Input: part model. Units: mm. Frame: model coordinates. Face numbers are marked on the shaded views. A direction names the side the tool comes from. Coordinates: 2 decimals unless noted, no trailing zeros. Order: outer loops, then holes, each group sorted by start corner. A loop starts at its lowest first (then second) coordinate and runs counter-clockwise, first axis right, second up. Notation, with made-up numbers: (38, -21.5) - (46, -21.5) arc R27 ccw to (46, 5.5) - close; hole circle Ø2 at (33.25, -26). An arc over 180 degrees is marked (long way). Use a Markdown table: item, result. Add a question column.
from build123d import *

# Parameters (mm, degrees)
SKETCH1_R           = 4
BOSS_EXTRUDE1_DEPTH = 1
SKETCH2_R           = 3
BOSS_EXTRUDE2_DEPTH = 2
FILLET1_R           = 1
SKETCH3_R           = 2
CUT_EXTRUDE1_DEPTH  = 4
FILLET2_R           = 1


with BuildPart() as part:
    # Sketch1 → Boss-Extrude1 (new body)
    with BuildSketch(Plane.XY):
        Circle(SKETCH1_R)
    extrude(amount=BOSS_EXTRUDE1_DEPTH)

    # Sketch2 → Boss-Extrude2 (add)
    with BuildSketch(Plane.XY.offset(1)):
        Circle(SKETCH2_R)
    extrude(amount=BOSS_EXTRUDE2_DEPTH)

    # Fillet1
    fillet1_edges = [part.edges().sort_by_distance(p)[0] for p in [
        (-3, 0, 1),
    ]]
    fillet(fillet1_edges, radius=FILLET1_R - 0.0001)  # a hair under: the kernel refuses the full size

    # Sketch3 → Cut-Extrude1 (cut)
    with BuildSketch(Plane.XY.offset(3)):
        Circle(SKETCH3_R)
    extrude(amount=-CUT_EXTRUDE1_DEPTH, mode=Mode.SUBTRACT)

    # Fillet2
    fillet2_edges = [part.edges().sort_by_distance(p)[0] for p in [
        (-2, 0, 0),
    ]]
    fillet(fillet2_edges, radius=FILLET2_R)


solid = part.part
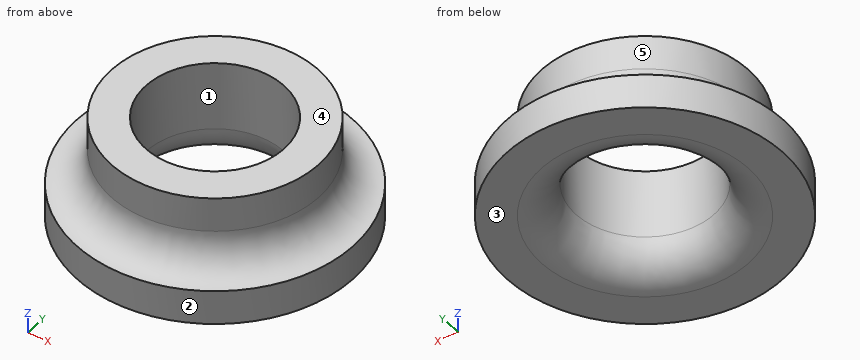
1) Cut plane D-D (z = 0.4). Return the cut outline in (x, y), and give its area (3 significant figures).
2) Contact query for a flat-ended pin moving along its axis: P1, Ø4.5, axis at x = 0, y = 0, coming from the -Z side. Output: stop coordinate, or through.
3) Cut plane C-C (z = 2.4). Return the cut outline in (x, y), and give its area (3 significant figures).
4) Pull-direction query (X, two-part tool) for the marked faces 1, 2 and 3; classes: pulls with the +X half, pulls with the -X half, needs draft (parallel to the pull), parting line crosses it, or undercut.
5) Reachability of the marked faces 4 and 5 from +Z, -Z, +X, -X, +Y, -Y: full face, straight path, thin tool, end or side. Return the list, or none.
6) Material intervals for L1, parallel to Y at x = 0, z = 1.95; L2, parallel to Y at x = -1.75, z = 1.5; L3, parallel to X at y = 0.5, z = 1.25, sorted ascending.
Computed:
| question | item | result |
|---|---|---|
| 1 | outline | circle Ø8 at (0, 0); hole circle Ø4.4 at (0, 0) |
| 1 | area | 35.1 mm2 |
| 2 | P1 | stops at z = 0.34 |
| 3 | outline | circle Ø6 at (0, 0); hole circle Ø4 at (0, 0) |
| 3 | area | 15.7 mm2 |
| 4 | face 1 | undercut |
| 4 | face 2 | parting line crosses it |
| 4 | face 3 | needs draft |
| 5 | face 4 | +Z, +X, -X, +Y, -Y |
| 5 | face 5 | +Z |
| 6 | L1 | y = -3 to -2, 2 to 3 |
| 6 | L2 | y = -2.6 to -0.97, 0.97 to 2.6 |
| 6 | L3 | x = -3.3 to -1.94, 1.94 to 3.3 |
